Here's how the part is built. I have some questions about the finished solid (model axes, mm). A direction names the side the tool comes from. Round coordinates to 2 decimals unless told otherwise and drop trailing zeros. Order: outer loops, then holes, each group sorted by start corner. A loop starts at its lowest first (then second) coordinate and runs counter-clockwise, first axis right, second up. Notation, with made-up numbers: (-19.5, 49.25) -> (-7.5, 49.25) arc R16 cw to (-7.5, 53.25) -> close; hole circle Ø6 at (-31.75, 85). An arc over 180 degrees is marked (long way). Use a Markdown table: item, result. Add a question column.
(1) I want a section at B-B, the plane x = -354.5. Please give me the cut outline in (y, z), then the cut area to 3 significant figures.
(2) If I drill on probe 1 along X at (y, z) = (363, -218.5); probe 2 along X at (y, z) = (411, -169.5), over which ranges is the centre line in solid material (lowest first)?
(3) On a 3-axis mill with a long thin cutter (end or side, diameter ignored), from which of +Z, -Z, +X, -X, +Y, -Y can I reach the whole of each face in a straight line? I mean faces 4 (the face through (-347.376, 358.435, -220.958)), 5 (the face through (-340.067, 370.937, -238.256)). Say none if no direction works.
(4) I want a section at A-A, the plane y = 370. Give the number of separate pieces and of enclosed holes in the cut face, then the cut area to 3 significant figures.
(5) Thinking about a two-plate mould opening in Y: for faces 1 (the face through (-332.74, 393.85, -220.86)), 2 (the face through (-321.905, 431.021, -200.914)), 3 (the face through (-329.002, 400.258, -235.664)), which applies, pulls with the +Y half, pulls with the -Y half, needs draft (parallel to the pull), parting line crosses it, or undercut?
(6) I want a section at C-C, the plane z = -160. Please give me the cut outline in (x, y), then the cut area to 3 significant figures.
(7) I'm going to push flat-ended pins straight in: P1, Ø12, axis at y = 408, z = -175, coming from the +X side; P2, Ø6, axis at y = 414.5, z = -216, coming from the +X side; P3, Ø12, axis at y = 409, z = -235, coming from the -X side. Where does each tip first touch, or does it pass through?
from build123d import *

# Parameters (mm, degrees)
SKETCH39_R          = 11.25
SKETCH39_R_2        = 3.55
SKETCH39_R_3        = 4.024999951
BOSS_EXTRUDE1_DEPTH = 1.5875


with BuildPart() as part:
    # Sketch39 → Boss-Extrude1 (new body)
    with BuildSketch(Plane(origin=(-441.521969452, 172.104793819, -62.182961286), x_dir=(-0.12122181659134341, 0.04725213510134498, 0.9915001295565519), z_dir=(-0.9237984742451071, 0.3600956621414251, -0.1301056996804562))):
        with BuildLine():
            Line((-227.779978176, 213.473332746), (-90.363815922, 201.963804234))
            Line((-90.363815922, 201.963804234), (-90.363815922, 280.537968932))
            Line((-90.363815922, 280.537968932), (-190.676741831, 288.939851665))
            ThreePointArc((-190.676741831, 288.939851665), (-213.041445426, 281.797087727), (-223.80498218, 260.932157339))
            Line((-223.80498218, 260.932157339), (-227.779978176, 213.473332746))
        make_face()
        with Locations(Location((-128.463815922, 252.946692942, 0), (0, 0, 270))):
            Circle(SKETCH39_R, mode=Mode.SUBTRACT)
        with Locations(Location((-108.73290302, 251.294096181, 0), (0, 0, 270))):
            Circle(SKETCH39_R_2, mode=Mode.SUBTRACT)
        with Locations(Location((-148.194728824, 254.599289703, 0), (0, 0, 270))):
            Circle(SKETCH39_R_2, mode=Mode.SUBTRACT)
        with Locations(Location((-193.237014843, 258.371884328, 0), (0, 0, 270))):
            Circle(SKETCH39_R, mode=Mode.SUBTRACT)
        with Locations(Location((-173.506101941, 256.719287567, 0), (0, 0, 270))):
            Circle(SKETCH39_R_2, mode=Mode.SUBTRACT)
        with Locations(Location((-212.967927745, 260.024481088, 0), (0, 0, 270))):
            Circle(SKETCH39_R_2, mode=Mode.SUBTRACT)
        with Locations(Location((-131.378812986, 218.143554906, 0), (0, 0, 270))):
            Circle(SKETCH39_R_3, mode=Mode.SUBTRACT)
        with BuildLine():
            Line((-210.812041783, 230.315880525), (-205.885245836, 229.903228203))
            ThreePointArc((-205.885245836, 229.903228203), (-202.798738622, 224.125454392), (-206.803355147, 218.941609924))
            Line((-206.803355147, 218.941609924), (-211.730151094, 219.354262246))
            ThreePointArc((-211.730151094, 219.354262246), (-214.816658309, 225.132036057), (-210.812041783, 230.315880525))
        make_face(mode=Mode.SUBTRACT)
        with BuildLine():
            Line((-185.500668667, 228.195882655), (-180.57387272, 227.783230333))
            ThreePointArc((-180.57387272, 227.783230333), (-177.48736551, 222.005456528), (-181.49198203, 216.821612065))
            Line((-181.49198203, 216.821612065), (-186.418777977, 217.234264387))
            ThreePointArc((-186.418777977, 217.234264387), (-189.505285187, 223.012038192), (-185.500668667, 228.195882655))
        make_face(mode=Mode.SUBTRACT)
    extrude(amount=BOSS_EXTRUDE1_DEPTH)


solid = part.part
Taken from the geometry:
| question | item | result |
|---|---|---|
| 1 | outline | (356.56, -169.55) -> (357.43, -179.35) -> (367.32, -151.99) -> (362.98, -151.78) -> close |
| 1 | area | 99.5 mm2 |
| 2 | probe 1 | x = -346.81 to -345.1 |
| 2 | probe 2 | x = -335.01 to -333.29 |
| 3 | face 4 | -Z, -X, -Y |
| 3 | face 5 | none |
| 4 | separate pieces | 4 |
| 4 | enclosed holes | 0 |
| 4 | area | 180 mm2 |
| 5 | face 1 | pulls with the -Y half |
| 5 | face 2 | pulls with the +Y half |
| 5 | face 3 | undercut |
| 6 | outline | (-357.46, 356.83) -> (-355.96, 356.26) -> (-327.42, 429.47) -> (-328.92, 430.04) -> close |
| 6 | area | 126 mm2 |
| 7 | P1 | stops at x = -331.19 |
| 7 | P2 | stops at x = -324.13 |
| 7 | P3 | stops at x = -328.86 |
